The listing builds one solid part. Answer for the finished solid, in the listing's coordinates (mm). Face numbers are marked on the shaded views. A direction names the side the tool comes from. Round coordinates to 2 decimals unless told otherwise and drop trailing zeros. Write each loop counter-clockwise with the first axis right and the second up, starting at its lowest first coordinate (ties: lowest second). Pieces come first, ordered by that corner, then holes.
(1) Find the intervals of material crossed by probe 1 along X at (y, z) = (-9.25, 12); probe 2 along X at (y, z) = (4.75, 18.5); probe 3 along Y at (x, z) = (-20, 3), in increasing order.
(2) A cutting plane is placed at A-A, the plane y = -7.5. Give the vertices of the cut face in (x, z), and give its area (3 significant figures).
(3) A cutting plane is placed at B-B, the plane x = -19. Give the vertices of the cut face in (y, z).
(4) Each of these flat-tipped pins is pushed along its axis until it touches: pin 1 Ø10 at (x, y) = (-10, 1.5) entering from -Z; pin 2 Ø6.5 at (y, z) = (0, 38.5) entering from +X; pin 3 Ø5 at (x, z) = (15, 40.5) entering from +Y; pin 4 Ø10 at (x, z) = (-4.5, 43) entering from -Y. Where does it stop, or does it pass through?
(5) For the marked faces 1, 2, 3, 4 and 5, determine the directions among +Z, -Z, +X, -X, +Y, -Y from which every point of the face is accessible in a straight line to the end or side of a thin tool.
(6) The mould has two halves that part along X. Classify the marked faces 6, 7 and 8: +X half, -X half, draft (parallel to the pull), parting line (faces both ways), or undercut.
(7) A cutting plane is placed at D-D, the plane y = 0.5. Give the vertices of the cut face in (x, z), and give its area (3 significant figures).
(8) A cutting plane is placed at C-C, the plane z = 20. Give the vertices of the cut face in (x, y), and give its area (3 significant figures).
from build123d import *

# Parameters (mm, degrees)
F0_W     = 46
F0_H     = 22
F1_DEPTH = 30
F2_W     = 41
F2_H     = 17
F3_DEPTH = 22
F4_W     = 36
F4_H     = 22
F5_DEPTH = 4
F6_W     = 22
F6_H     = 6
F7_DEPTH = 20


with BuildPart() as f1:
    # F0 (on Top) → F1 (new body)
    with BuildSketch(Plane.XY):
        Rectangle(F0_W, F0_H)
    extrude(amount=F1_DEPTH)

    # F2 (on face) → F3 (cut)
    with BuildSketch(Plane(origin=(0, 0, 0), x_dir=(1, 0, 0), z_dir=(0, 0, -1))):
        Rectangle(F2_W, F2_H)
    extrude(amount=-F3_DEPTH, mode=Mode.SUBTRACT)

    # F4 (on face) → F5 (cut)
    with BuildSketch(Plane.XZ.offset(11)):
        with Locations((0, 11)):
            Rectangle(F4_W, F4_H)
    extrude(amount=-F5_DEPTH, mode=Mode.SUBTRACT)

    # F6 (on face) → F7 (join)
    with BuildSketch(Plane.XY.offset(30)):
        Rectangle(F6_W, F6_H)
    extrude(amount=F7_DEPTH)


solid = f1.part
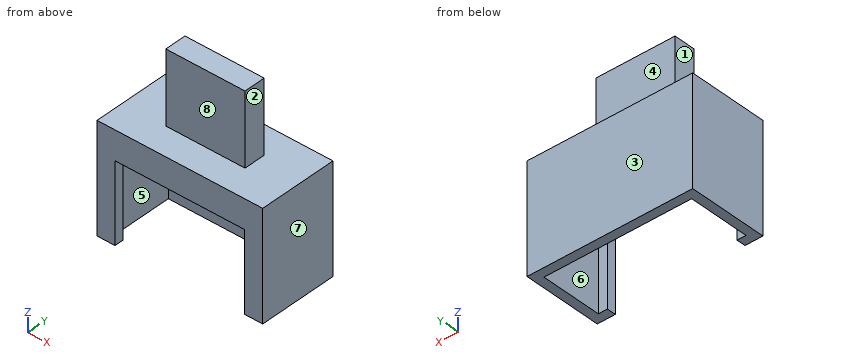
Solutions:
1. probe 1: x = -23 to -18, 18 to 23
1. probe 2: x = -23 to -20.5, 20.5 to 23
1. probe 3: y = -11 to -8.5, 8.5 to 11
2. outline: (-23, 0) - (-20.5, 0) - (-20.5, 22) - (20.5, 22) - (20.5, 0) - (23, 0) - (23, 30) - (-23, 30) - close
2. area: 478 mm2
3. outline: (-11, 0) - (-8.5, 0) - (-8.5, 22) - (8.5, 22) - (8.5, 0) - (11, 0) - (11, 30) - (-11, 30) - close
4. pin 1: stops at z = 22
4. pin 2: stops at x = 11
4. pin 3: passes through
4. pin 4: stops at y = -3
5. face 1: +Z, -X, +Y, -Y
5. face 2: +Z, +X, +Y, -Y
5. face 3: +Z, -Z, +X, -X, +Y
5. face 4: +Z, +X, -X, +Y
5. face 5: -Z
6. face 6: undercut
6. face 7: +X half
6. face 8: draft
7. outline: (-23, 0) - (-20.5, 0) - (-20.5, 22) - (20.5, 22) - (20.5, 0) - (23, 0) - (23, 30) - (11, 30) - (11, 50) - (-11, 50) - (-11, 30) - (-23, 30) - close
7. area: 918 mm2
8. outline: (-23, -11) - (-18, -11) - (-18, -8.5) - (-20.5, -8.5) - (-20.5, 8.5) - (20.5, 8.5) - (20.5, -8.5) - (18, -8.5) - (18, -11) - (23, -11) - (23, 11) - (-23, 11) - close
8. area: 225 mm2
